from build123d import *

# Parameters (mm, degrees)
SKETCH_1_R          = 13
SKETCH_1_R_2        = 10.825
RING_DEPTH          = 5
SKETCH_2_W          = 50
SKETCH_2_H          = 8
STICK_DEPTH         = 5
SKETCH_3_W          = 21
SKETCH_3_H          = 8
KEY_DEPTH           = 10
FILLET_1_R          = 5
FILLET_5_R          = 2
KEY_HOLE_DEPTH      = 64.037665059
KEY_HOLE_DEPTH_BACK = 64.037665059
CUT_EXTRUDE_2_DEPTH = 64.3837299


with BuildPart() as part:
    # Эскиз1 → ring (new body)
    with BuildSketch(Plane(origin=(0, 0, 0), x_dir=(1, 0, 0), z_dir=(0, 1, 0))):
        with Locations(Location((0, 0, 0), (0, 0, 270))):
            Circle(SKETCH_1_R)
        with Locations(Location((0, 0, 0), (0, 0, 270))):
            Circle(SKETCH_1_R_2, mode=Mode.SUBTRACT)
    extrude(amount=RING_DEPTH)

    # Эскиз2 → stick (add)
    with BuildSketch(Plane(origin=(0, 0, 0), x_dir=(1, 0, 0), z_dir=(0, 1, 0))):
        with Locations((-36.22497216, -1.5)):
            Rectangle(SKETCH_2_W, SKETCH_2_H)
    extrude(amount=STICK_DEPTH)

    # Эскиз3 → key (add)
    with BuildSketch(Plane(origin=(0, 0, 0), x_dir=(1, 0, 0), z_dir=(0, 1, 0))):
        with Locations((-50.72497216, -1.5)):
            Rectangle(SKETCH_3_W, SKETCH_3_H)
    extrude(amount=KEY_DEPTH)

    # Скругление1
    fillet_1_edges = [part.edges().sort_by_distance(p)[0] for p in [
        (-11.779218989, 2.5, 5.5),
        (-12.757350822, 2.5, -2.5),
    ]]
    fillet(fillet_1_edges, radius=FILLET_1_R)

    # Скругление5
    fillet_5_edges = [part.edges().sort_by_distance(p)[0] for p in [
        (-40.22497216, 5, 1.5),
    ]]
    fillet(fillet_5_edges, radius=FILLET_5_R)

    # Эскиз4 → key hole (cut, two sides: drawn at the far end of the back side and taken through both)
    with BuildSketch(Plane(origin=(0, 2.5, 0), x_dir=(1, 0, 0), z_dir=(0, 1, 0)).offset(-KEY_HOLE_DEPTH_BACK)):
        Polygon((-61.22497216, -1), (-41.22497216, -1), (-41.22497216, -2), (-42.388207879, -2), (-42.82497216, -3.2), (-44.62497216, -3.2), (-45.061736441, -2), (-46.22497216, -2), (-47.388207879, -2), (-47.82497216, -3.2), (-49.62497216, -3.2), (-50.061736441, -2), (-51.22497216, -2), (-52.388207879, -2), (-52.82497216, -3.2), (-54.62497216, -3.2), (-55.061736441, -2), (-56.22497216, -2), (-57.388207879, -2), (-57.82497216, -3.2), (-59.62497216, -3.2), (-60.061736441, -2), (-61.22497216, -2), align=None)
    extrude(amount=KEY_HOLE_DEPTH + KEY_HOLE_DEPTH_BACK, mode=Mode.SUBTRACT)

    # Эскиз5 → Вытянуть2 (cut, through all)
    with BuildSketch(Plane.XZ):
        Polygon((-25.2, -2.5), (-25.2, 0), (0, 0), (0, -0.2), (-25, -0.2), (-25, -2.5), align=None)
    extrude(amount=-CUT_EXTRUDE_2_DEPTH, mode=Mode.SUBTRACT)


solid = part.part
The model under review builds one solid part; all positions refer to its coordinate system, in mm. A direction names the side the tool comes from. Round coordinates to 2 decimals unless told otherwise and drop trailing zeros. Order: outer loops, then holes, each group sorted by start corner. A loop starts at its lowest first (then second) coordinate and runs counter-clockwise, first axis right, second up. Notation, with made-up numbers: (74, 52.5) - (110, 52.5) arc R9 ccw to (110, 66.5) - close; hole circle Ø10 at (53, 34). An arc over 180 degrees is marked (long way). Use one line per item in the form item = value.
Q1. Clearance check with flat-ended pins moving along their axes: P1, Ø2.5, axis at x = -56, y = 6, coming from the -Z side; P2, Ø1.5, axis at y = 9, z = 2.5, coming from the +X side (3 decimals); P3, Ø3, axis at x = -50.5, y = 4.5, coming from the +Z side; P4, Ø12, axis at x = -36.5, z = 8, coming from the +Y side. State where each tip first meets the part, or that it passes through.
Response values:
P1 = -2.5
P2 = -40.225
P3 = 5.5
P4 = 10
Q2. Tool access review of faces 1 (the flat face through (-18, 2, 0)), 2 (the flat face through (-56, 5, 2)), 3 (the flat face through (-21, 2, -2.5)), 4 (the flat face through (-43, 4, 5.5)), 5 (the flat face through (-15, 5, 2)): name each direction out of +Z, -Z, +X, -X, +Y, -Y from which nothing blocks a thin tool from reaching the whole face with its end or side.
Response values:
face_1 = +Y, -Y
face_2 = -X, +Y, -Y
face_3 = -Z, -X, +Y, -Y
face_4 = +Z, -X, +Y, -Y
face_5 = +Z, -Z, +X, +Y
Q3. Add section A-A on x = -48.5. Give the boundary of the cut face in (y, z).
Response values:
outline = (0, -2.5) - (10, -2.5) - (10, 1) - (0, 1) - close; (0, 3.2) - (10, 3.2) - (10, 5.5) - (0, 5.5) - close
Q4. To check wall thickness, follow line 1 (Z direction, x = 0, y = 3.6) (3 decimals); line 2 (Z direction, x = -57, y = 4); line 3 (X direction, y = 1, z = -1.75). State the ranges of each line that lie inside material, in increasing order.
Response values:
line_1 = -13 to -10.825, 10.825 to 13
line_2 = -2.5 to 1, 2 to 5.5
line_3 = -61.22 to -25.2, -25 to -10.68, 10.68 to 12.88
Q5. Add section B-B on y = 9.25. Give the boundary of the cut face in (x, z), then the cut area to 3 significant figures.
Response values:
outline = (-61.22, -2.5) - (-40.22, -2.5) - (-40.22, 5.5) - (-61.22, 5.5) - (-61.22, 2) - (-60.06, 2) - (-59.62, 3.2) - (-57.82, 3.2) - (-57.39, 2) - (-55.06, 2) - (-54.62, 3.2) - (-52.82, 3.2) - (-52.39, 2) - (-50.06, 2) - (-49.62, 3.2) - (-47.82, 3.2) - (-47.39, 2) - (-45.06, 2) - (-44.62, 3.2) - (-42.82, 3.2) - (-42.39, 2) - (-41.22, 2) - (-41.22, 1) - (-61.22, 1) - close
area = 137 mm^2
Q6. Add section D-D on x = -1.5. Give the boundary of the cut face in (y, z), then the cut area to 3 significant figures.
Response values:
outline = (0, -12.91) - (5, -12.91) - (5, -10.72) - (0, -10.72) - close; (0, 10.72) - (5, 10.72) - (5, 12.91) - (0, 12.91) - close
area = 21.9 mm^2
Q7. Add section C-C on z = 4. Give the boundary of the cut face in (x, y).
Response values:
outline = (-61.22, 0) - (-10.06, 0) - (-10.06, 5) - (-38.22, 5) arc R2 cw to (-40.22, 7) - (-40.22, 10) - (-61.22, 10) - close; (10.06, 0) - (12.37, 0) - (12.37, 5) - (10.06, 5) - close
Q8. Mouldability with a two-part tool opening along X and no side actions: class faces 6 (the flat face through (-59, 5, 3.2)), 7 (the flat face through (-51, 5, 2)), 8 (the flat face through (-61.225, 5, -1)), 9 (the flat face through (-44.84, 4.93, 2.61)) as pulls with the +X half, pulls with the -X half, needs draft (parallel to the pull), parting line crosses it, or undercut.
Response values:
face_6 = undercut
face_7 = needs draft
face_8 = pulls with the -X half
face_9 = undercut
